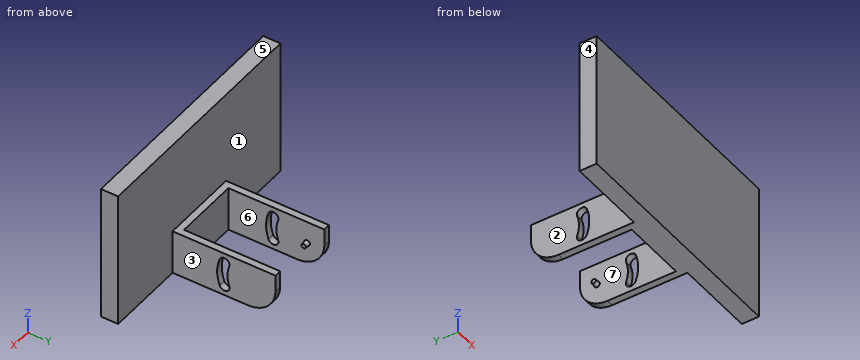
from build123d import *

# Parameters (mm, degrees)
SKETCH2_W               = 19.1
SKETCH2_H               = 13
BOSS_EXTRUDE1_DEPTH     = 2
BOSS_EXTRUDE2_DEPTH     = 2
SKETCH4_R               = 0.8
BOSS_EXTRUDE3_DEPTH     = 1.5
BOSS_EXTRUDE3_TAPER     = 5
CUT_EXTRUDE1_DEPTH      = 38.248624136
CUT_EXTRUDE1_DEPTH_BACK = 38.248624136
SKETCH6_W               = 70
SKETCH6_H               = 40
BOSS_EXTRUDE4_DEPTH     = 5


with BuildPart() as part:
    # Sketch2 → Boss-Extrude1 (new body)
    with BuildSketch(Plane(origin=(0, 0, 0), x_dir=(1, 0, 0), z_dir=(0, 1, 0))):
        Rectangle(SKETCH2_W, SKETCH2_H)
    extrude(amount=BOSS_EXTRUDE1_DEPTH)

    # Sketch3 → Boss-Extrude2 (add)
    with BuildSketch(Plane.ZY.offset(9.55)):
        with BuildLine():
            Line((6.5, 0), (6.5, 30))
            Line((6.5, 30), (1.5, 30))
            ThreePointArc((1.5, 30), (-4.156854249, 27.656854249), (-6.5, 22))
            Line((-6.5, 22), (-6.5, 0))
            Line((-6.5, 0), (6.5, 0))
        make_face()
    boss_extrude2 = extrude(amount=BOSS_EXTRUDE2_DEPTH)

    # Sketch4 → Boss-Extrude3 (add)
    with BuildSketch(Plane(origin=(-9.55, 0, 0), x_dir=(0, 0, -1), z_dir=(1, 0, 0))):
        with Locations((0, 25)):
            Circle(SKETCH4_R)
    boss_extrude3 = extrude(amount=BOSS_EXTRUDE3_DEPTH, taper=BOSS_EXTRUDE3_TAPER)

    # Mirror1: Boss-Extrude2, Boss-Extrude3 across plane
    add(boss_extrude2.mirror(Plane(origin=(0, 0, 0), x_dir=(0, 0, 1), z_dir=(1, 0, 0))))
    add(boss_extrude3.mirror(Plane(origin=(0, 0, 0), x_dir=(0, 0, 1), z_dir=(1, 0, 0))))

    # Sketch5 → Cut-Extrude1 (cut, two sides: drawn at the far end of the back side and taken through both)
    with BuildSketch(Plane(origin=(-9.55, 0, 0), x_dir=(0, 0, -1), z_dir=(1, 0, 0)).offset(-CUT_EXTRUDE1_DEPTH_BACK)):
        with BuildLine():
            ThreePointArc((3.07818129, 16.542766413), (5.000750436, 15.646257697), (4.10424172, 13.723688551))
            ThreePointArc((4.10424172, 13.723688551), (0, 13), (-4.10424172, 13.723688551))
            ThreePointArc((-4.10424172, 13.723688551), (-5.000750436, 15.646257697), (-3.07818129, 16.542766413))
            ThreePointArc((-3.07818129, 16.542766413), (0, 16), (3.07818129, 16.542766413))
        make_face()
    extrude(amount=CUT_EXTRUDE1_DEPTH + CUT_EXTRUDE1_DEPTH_BACK, mode=Mode.SUBTRACT)

    # Sketch6 → Boss-Extrude4 (add)
    with BuildSketch(Plane.XZ):
        with Locations((0, 13.5)):
            Rectangle(SKETCH6_W, SKETCH6_H)
    extrude(amount=BOSS_EXTRUDE4_DEPTH)


solid = part.part
The listing builds one solid part. Answer for the finished solid, in the listing's coordinates (mm). Face numbers are marked on the shaded views. A direction names the side the tool comes from. Coordinates: 2 decimals unless noted, no trailing zeros. Write each loop counter-clockwise with the first axis right and the second up, starting at its lowest first coordinate (ties: lowest second). Pieces come first, ordered by that corner, then holes. Notation, with made-up numbers: M 83.25,-15.75 L 136.25,-15.75 A20 ccw 136.25,20.25 Z; hole C 39.25,69 d5. An arc over 180 degrees is marked long. Write each question's results on one line, items separated by ' | '.
Item 1: Given P1, Ø5, axis at x = -11, y = 6.5, coming from the +Z side; P2, Ø8, axis at x = -7.5, z = 16, coming from the +Y side; P3, Ø4, axis at y = 17, z = -1, coming from the +X side, each flat-ended and moving along its own axis, determine where each tip first touches the part or whether it passes through.
Answer below:
P1: z = 6.5 | P2: y = 0 | P3: x = 11.55
Item 2: The part is cut by section B-B on z = 14.5. Determine the outline of the cut face in (x, y).
Answer below:
outline: M -35,-5 L 35,-5 L 35,0 L -35,0 Z
Item 3: The part is cut by section A-A on y = 20. Determine the outline of the cut face in (x, z).
Answer below:
outline: M -11.55,-6.5 L -9.55,-6.5 L -9.55,6.5 L -11.55,6.5 Z; M 9.55,-6.5 L 11.55,-6.5 L 11.55,6.5 L 9.55,6.5 Z
Item 4: Which of the six approach directions +Z, -Z, +X, -X, +Y, -Y give full straight-line access (tool end or side, diameter ignored) to the marked faces 1, 2 and 3?
Answer below:
face 1: +Z, +Y | face 2: +Z, -Z, -X, +Y | face 3: +Z, -Z, +X, +Y
Item 5: Consider probe 1 along X at (y, z) = (23, 4); probe 2 along Z at (x, y) = (-11, 2). Determine where each line is inside the solid, lowest interval first. Write a range as [from, to].
Answer below:
probe 1: [-11.55, -9.55], [9.55, 11.55] | probe 2: [-6.5, 6.5]
Item 6: For a pull along X with two mould halves and no side action, classify the marked faces 4, 5, 6 and 7 as released by +X, released by -X, zero draft, split by the parting line, or undercut.
Answer below:
face 4: released by -X | face 5: zero draft | face 6: undercut | face 7: undercut
Item 7: The part is cut by section C-C on x = -18.5. Determine the outline of the cut face in (y, z), and give its area (3 significant figures).
Answer below:
outline: M -5,-6.5 L 0,-6.5 L 0,33.5 L -5,33.5 Z | area: 200 mm2
